Could you check a few things on this drawing? It's one solid part, dimensions in mm from its lowest x, y, z. A direction names the side the tool comes from. Give positions to 0.01 mm unless a question says otherwise; leave off trailing zeros. Order: outer loops, then holes, each group sorted by start corner. A loop starts at its lowest first (then second) coordinate and runs counter-clockwise, first axis right, second up.
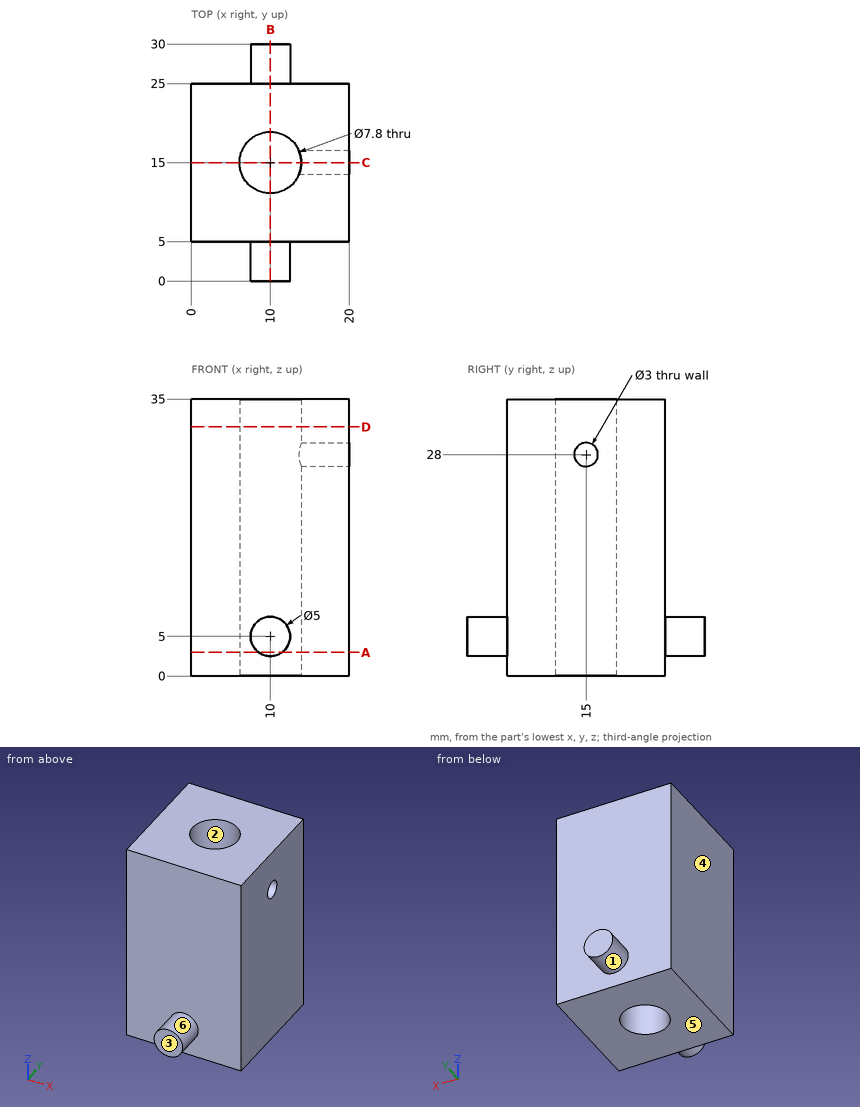
1) We'd pull the mould along X, two halves only. Please class the marked faces 1, 2, 3 and 4: +X half, -X half, draft (parallel to the pull), parting line (faces both ways), or undercut.
2) Which directions (+Z, -Z, +X, -X, +Y, -Y) give clear straight access to the entire face, cutting with the end or side of a thin tool? Please do the marked faces 5 and 6.
3) Suppose I cut it at D-D (z = 31.5). Please give me the cut outline in (x, y).
4) I'm going to push flat-ended pins straight in: pin 1 Ø3 at (x, z) = (3.5, 20.5) entering from +Y; pin 2 Ø2 at (x, z) = (10, 21) entering from -Y; pin 3 Ø8 at (y, z) = (11, 22) entering from -X; pin 4 Ø1.8 at (y, z) = (15, 28) entering from +X. Where does each tip first touch, or does it pass through?
5) If I drill on line 1 (X direction, y = 15, z = 20.5); line 2 (Z direction, x = 16.75, y = 15); line 3 (Y direction, x = 12.5, z = 24), over which ranges is the centre line in solid material (lowest first)?
6) Suppose I cut it at C-C (y = 15). Please give me the cut outline in (x, z), and give its area (3 significant figures).
7) Suppose I cut it at B-B (x = 10). Please give me the cut outline in (y, z).
8) Suppose I cut it at A-A (z = 3). Please give me the cut outline in (x, y).
Results:
1. face 1: parting line
1. face 2: undercut
1. face 3: draft
1. face 4: -X half
2. face 5: -Z, +X, -X, +Y, -Y
2. face 6: -Y
3. outline: (0, 5) - (20, 5) - (20, 25) - (0, 25) - close; hole circle Ø7.8 at (10, 15)
4. pin 1: stops at y = 25
4. pin 2: stops at y = 5
4. pin 3: stops at x = 0
4. pin 4: stops at x = 6.21
5. line 1: x = 0 to 6.1, 13.9 to 20
5. line 2: z = 0 to 26.5, 29.5 to 35
5. line 3: y = 5 to 12.01, 17.99 to 25
6. outline: (0, 0) - (6.1, 0) - (6.1, 35) - (0, 35) - close; (13.9, 0) - (20, 0) - (20, 26.5) - (13.9, 26.5) - close; (13.9, 29.5) - (20, 29.5) - (20, 35) - (13.9, 35) - close
6. area: 409 mm2
7. outline: (0, 2.5) - (5, 2.5) - (5, 0) - (11.1, 0) - (11.1, 35) - (5, 35) - (5, 7.5) - (0, 7.5) - close; (18.9, 0) - (25, 0) - (25, 2.5) - (30, 2.5) - (30, 7.5) - (25, 7.5) - (25, 35) - (18.9, 35) - close
8. outline: (0, 5) - (8.5, 5) - (8.5, 0) - (11.5, 0) - (11.5, 5) - (20, 5) - (20, 25) - (11.5, 25) - (11.5, 30) - (8.5, 30) - (8.5, 25) - (0, 25) - close; hole circle Ø7.8 at (10, 15)
